Part model, mm, in its own coordinate system. A direction names the side the tool comes from. Round coordinates to 2 decimals unless told otherwise and drop trailing zeros. Loops run counter-clockwise (first coordinate to the right, second up) from the corner with the lowest first, then second, coordinate; pieces in that order, holes last.
1) Band-saw the part on A-A, the plane y = 15. Write the cut outline in (x, z).
2) Mould opens along X. For faces 4 (the flat face through (45, -22, 1)), 5 (the flat face through (-65, 40, 2)) say: +X half, -X half, draft (parallel to the pull), parting line (faces both ways), or undercut.
3) Probe line 1 (X direction, y = -15, z = 1.9); line 2 (Y direction, x = 55, z = 1.6); line 3 (X direction, y = -24.5, z = 3.75). List the from-to ranges inside material, lowest first.
4) Band-saw the part on D-D, the plane x = 21.5. Write the cut outline in (y, z), then the cut area to 3 significant figures.
5) Drop flat-ended pins along their axis: P1, Ø3, axis at x = 6, z = 3.5, coming from the +Y side; P2, Ø5, axis at y = 23.5, z = 8, coming from the +X side; P3, Ø1, axis at x = 41, y = 9.5, coming from the +Z side; P4, Ø10, axis at x = 51, y = 8, coming from the +Z side. Give the stop position or say it passes through.
6) Band-saw the part on B-B, the plane y = -7. Write the cut outline in (x, z).
7) Band-saw the part on C-C, the plane x = 55. Write the cut outline in (y, z).
8) 3-axis set-ups, long thin cutter, end or side, ignore diameter. For faces 1 (the flat face through (-40, -26, 2)), 2 (the flat face through (-65, -5.046, 1)), 3 (the flat face through (-3, 9.5, 4)): which of +Z, -Z, +X, -X, +Y, -Y reach the whole face in a straight line?
from build123d import *

# Parameters (mm, degrees)
SKETCH_W        = 81
SKETCH_H        = 19
PAD_DEPTH       = 2.5
SKETCH001_W     = 82
SKETCH001_H     = 5
PAD001_DEPTH    = 2
SKETCH002_W     = 82
SKETCH002_H     = 5
PAD002_DEPTH    = 2
PAD003_DEPTH    = 2
POCKET_DEPTH    = 2
SKETCH005_W     = 50
SKETCH005_H     = 80
SKETCH005_W_2   = 30
PAD004_DEPTH    = 3
SKETCH006_R     = 2.48011
SKETCH006_R_2   = 2.438602
SKETCH006_R_3   = 2.48946
SKETCH006_W     = 5
SKETCH006_H     = 25
POCKET001_DEPTH = 3
SKETCH007_W     = 40
SKETCH007_H     = 5
POCKET002_DEPTH = 5
SKETCH008_W     = 2
SKETCH008_H     = 79.741493
SKETCH008_H_2   = 80
PAD005_DEPTH    = 1.5


with BuildPart() as part:
    # Sketch → Pad (new body)
    with BuildSketch(Plane.XY):
        Rectangle(SKETCH_W, SKETCH_H)
    extrude(amount=PAD_DEPTH)

    # Sketch001 (on Face3 of Pad) → Pad001 (join)
    with BuildSketch(Plane.XZ.offset(9.5)):
        with Locations((0, 2.5)):
            Rectangle(SKETCH001_W, SKETCH001_H)
    extrude(amount=PAD001_DEPTH)

    # Sketch002 (on Face11 of Pad001) → Pad002 (join)
    with BuildSketch(Plane(origin=(0, 9.5, 0), x_dir=(-1, 0, 0), z_dir=(0, 1, 0))):
        with Locations((0, 2.5)):
            Rectangle(SKETCH002_W, SKETCH002_H)
    extrude(amount=PAD002_DEPTH)

    # Sketch003 (on Face6 of Pad002) → Pad003 (join)
    with BuildSketch(Plane(origin=(0, 11.5, 0), x_dir=(-1, 0, 0), z_dir=(0, 1, 0))):
        with BuildLine():
            add(Edge.make_bspline(
                [(15, 2.06384), (20, 25), (25, 2.06384)],
                knots=[0, 0, 0, 1, 1, 1], degree=2))
            Line((25, 2.06384), (15, 2.06384))
        make_face()
    extrude(amount=-PAD003_DEPTH)

    # Sketch004 (on Face22 of Pad003) → Pocket (cut)
    with BuildSketch(Plane(origin=(0, 11.5, 0), x_dir=(-1, 0, 0), z_dir=(0, 1, 0))):
        with BuildLine():
            ThreePointArc((21.534306, 9.999999), (20, 11.534305), (18.465694, 9.999999))
            Line((18.465694, 9.999999), (18.465694, 3.999999))
            ThreePointArc((18.465694, 3.999999), (20, 2.465693), (21.534306, 3.999999))
            Line((21.534306, 9.999999), (21.534306, 3.999999))
        make_face()
    extrude(amount=-POCKET_DEPTH, mode=Mode.SUBTRACT)

    # Sketch005 (on Face5 of Pocket) → Pad004 (join)
    with BuildSketch(Plane(origin=(0, 0, 0), x_dir=(1, 0, 0), z_dir=(0, 0, -1))):
        with Locations((-65, 0)):
            Rectangle(SKETCH005_W, SKETCH005_H)
        with Locations((55, 0)):
            Rectangle(SKETCH005_W_2, SKETCH005_H)
    extrude(amount=-PAD004_DEPTH)

    # Sketch006 (on Face18 of Pad004) → Pocket001 (cut)
    with BuildSketch(Plane(origin=(0, 0, 0), x_dir=(1, 0, 0), z_dir=(0, 0, -1))):
        with Locations((55, -30)):
            Circle(SKETCH006_R)
        with Locations((55, -15)):
            Circle(SKETCH006_R_2)
        with Locations((55, 15)):
            Circle(SKETCH006_R_3)
        with Locations((55, 30)):
            Circle(SKETCH006_R_3)
        with Locations((62.5, 22.5)):
            Rectangle(SKETCH006_W, SKETCH006_H)
        with Locations((62.5, -22.5)):
            Rectangle(SKETCH006_W, SKETCH006_H)
        with Locations((47.5, -22.5)):
            Rectangle(SKETCH006_W, SKETCH006_H)
        with Locations((47.5, 22.5)):
            Rectangle(SKETCH006_W, SKETCH006_H)
    extrude(amount=-POCKET001_DEPTH, mode=Mode.SUBTRACT)

    # Sketch007 (on Face2 of Pocket001) → Pocket002 (cut)
    with BuildSketch(Plane(origin=(0, 0, 0), x_dir=(1, 0, 0), z_dir=(0, 0, -1))):
        with Locations((-65, 32.5)):
            Rectangle(SKETCH007_W, SKETCH007_H)
        with Locations((-65, 22.5)):
            Rectangle(SKETCH007_W, SKETCH007_H)
        with Locations((-65.12384, 7.546442)):
            Rectangle(SKETCH007_W, SKETCH007_H)
        with Locations((-65, -7.5)):
            Rectangle(SKETCH007_W, SKETCH007_H)
        with Locations((-65, -22.5)):
            Rectangle(SKETCH007_W, SKETCH007_H)
        with Locations((-65, -32.5)):
            Rectangle(SKETCH007_W, SKETCH007_H)
    extrude(amount=-POCKET002_DEPTH, mode=Mode.SUBTRACT)

    # Sketch008 (on Face47 of Pocket002) → Pad005 (join)
    with BuildSketch(Plane.XY.offset(3)):
        with Locations((41, -0.129254)):
            Rectangle(SKETCH008_W, SKETCH008_H)
        with Locations((-41, 0)):
            Rectangle(SKETCH008_W, SKETCH008_H_2)
    extrude(amount=PAD005_DEPTH)


solid = part.part
Reported:
1. outline: (-90, 0) - (-40, 0) - (-40, 4.5) - (-42, 4.5) - (-42, 3) - (-90, 3) - close; (40, 0) - (45, 0) - (45, 3) - (42, 3) - (42, 4.5) - (40, 4.5) - close; (50, 0) - (52.56, 0) - (52.56, 3) - (50, 3) - close; (57.44, 0) - (60, 0) - (60, 3) - (57.44, 3) - close; (65, 0) - (70, 0) - (70, 3) - (65, 3) - close
2. face 4: undercut
2. face 5: draft
3. line 1: x = -90 to -40, 40 to 45, 50 to 52.51, 57.49 to 60, 65 to 70
3. line 2: y = -40 to -32.49, -27.51 to -17.49, -12.51 to 12.56, 17.44 to 27.52, 32.48 to 40
3. line 3: x = -42 to -40, 40 to 42
4. outline: (-11.5, 0) - (11.5, 0) - (11.5, 5) - (9.5, 5) - (9.5, 2.5) - (-9.5, 2.5) - (-9.5, 5) - (-11.5, 5) - close
4. area: 67.5 mm2
5. P1: stops at y = 11.5
5. P2: passes through
5. P3: stops at z = 5
5. P4: stops at z = 3
6. outline: (-90, 0) - (-85.12, 0) - (-85.12, 3) - (-90, 3) - close; (-45.12, 0) - (70, 0) - (70, 3) - (42, 3) - (42, 4.5) - (40, 4.5) - (40, 2.5) - (-40, 2.5) - (-40, 4.5) - (-42, 4.5) - (-42, 3) - (-45.12, 3) - close
7. outline: (-40, 0) - (-32.49, 0) - (-32.49, 3) - (-40, 3) - close; (-27.51, 0) - (-17.49, 0) - (-17.49, 3) - (-27.51, 3) - close; (-12.51, 0) - (12.56, 0) - (12.56, 3) - (-12.51, 3) - close; (17.44, 0) - (27.52, 0) - (27.52, 3) - (17.44, 3) - close; (32.48, 0) - (40, 0) - (40, 3) - (32.48, 3) - close
8. face 1: +Z, -Z, -Y
8. face 2: +Z, -Z
8. face 3: +Z
